```python
from build123d import *

# Parameters (mm, degrees)
SKETCH1_R           = 37.5
BOSS_EXTRUDE1_DEPTH = 28.75
SKETCH2_R           = 31.5
SKETCH2_R_2         = 15.75
BOSS_EXTRUDE2_DEPTH = 6.5
SKETCH3_R           = 6
BOSS_EXTRUDE3_DEPTH = 58.85
SKETCH4_R           = 7.5
BOSS_EXTRUDE4_DEPTH = 4.7
CHAMFER1_SIZE       = 1
SKETCH5_R           = 2.5
CUT_EXTRUDE1_DEPTH  = 8
CHAMFER2_SIZE       = 1


with BuildPart() as part:
    # Sketch1 → Boss-Extrude1 (new body)
    with BuildSketch(Plane(origin=(0, 0, 0), x_dir=(1, 0, 0), z_dir=(0, 1, 0))):
        with Locations(Location((0, 0, 0), (0, 0, 90))):
            Circle(SKETCH1_R)
    extrude(amount=BOSS_EXTRUDE1_DEPTH)

    # Sketch2 → Boss-Extrude2 (add)
    with BuildSketch(Plane(origin=(0, 28.75, 0), x_dir=(1, 0, 0), z_dir=(0, 1, 0))):
        with Locations(Location((0, 0, 0), (0, 0, 90))):
            Circle(SKETCH2_R)
        with Locations(Location((0, 0, 0), (0, 0, 90))):
            Circle(SKETCH2_R_2, mode=Mode.SUBTRACT)
    extrude(amount=BOSS_EXTRUDE2_DEPTH)

    # Sketch3 → Boss-Extrude3 (add)
    with BuildSketch(Plane.XZ):
        with Locations(Location((0, 0, 0), (0, 0, 270))):
            Circle(SKETCH3_R)
    extrude(amount=BOSS_EXTRUDE3_DEPTH)

    # Sketch4 → Boss-Extrude4 (add)
    with BuildSketch(Plane.XZ):
        with Locations(Location((0, 0, 0), (0, 0, 90))):
            Circle(SKETCH4_R)
    extrude(amount=BOSS_EXTRUDE4_DEPTH)

    # Chamfer1
    chamfer1_edges = [part.edges().sort_by_distance(p)[0] for p in [
        (0, 28.75, 37.5),
        (0, 35.25, 31.5),
    ]]
    chamfer(chamfer1_edges, length=CHAMFER1_SIZE)

    # Sketch5 → Cut-Extrude1 (cut)
    with BuildSketch(Plane(origin=(0, 35.25, 0), x_dir=(1, 0, 0), z_dir=(0, 1, 0))):
        with Locations(Location((0, 25, 0), (0, 0, 270))):
            Circle(SKETCH5_R)
        with Locations(Location((25, 0, 0), (0, 0, 270))):
            Circle(SKETCH5_R)
        with Locations(Location((0, -25, 0), (0, 0, 270))):
            Circle(SKETCH5_R)
        with Locations(Location((-25, 0, 0), (0, 0, 270))):
            Circle(SKETCH5_R)
    extrude(amount=-CUT_EXTRUDE1_DEPTH, mode=Mode.SUBTRACT)

    # Chamfer2
    chamfer2_edges = [part.edges().sort_by_distance(p)[0] for p in [
        (0, 35.25, -27.5),
        (25, 35.25, -2.5),
        (0, 35.25, 22.5),
        (-25, 35.25, -2.5),
    ]]
    chamfer(chamfer2_edges, length=CHAMFER2_SIZE)


solid = part.part
```
Check sheet for the modelled part. Datum: model origin and axes. Units: mm. A direction names the side the tool comes from. Round coordinates to 2 decimals unless told otherwise and drop trailing zeros. Order: outer loops, then holes, each group sorted by start corner. A loop starts at its lowest first (then second) coordinate and runs counter-clockwise, first axis right, second up. Notation, with made-up numbers: (84.25, -33.75) -> (118.25, -33.75) arc R28 ccw to (118.25, -13.75) -> close; hole circle Ø7 at (41.25, -7). An arc over 180 degrees is marked (long way). Use CSV: the item, a comma, the result in double quotes.
(1) Depth check by flat-ended pin: pin 1 (2.5 mm diameter, centred on x = -26, z = -0.5, fed in from +Y); pin 2 (4 mm diameter, centred on x = 1, z = 25, fed in from +Y); pin 3 (19 mm diameter, centred on x = 0, z = 0, fed in from +Y). Enter the tip coordinate at first touch or a pass-through.
Worked out:
pin 1,"y = 27.25"
pin 2,"y = 34.75"
pin 3,"y = 28.75"
(2) Cross-section at A-A (y = -46). Record the boundary of the cut face in (x, z).
Worked out:
outline,"circle Ø12 at (0, 0)"
(3) Tool access check on faces 1 (the face through (-6, -4.7, 2)), 2 (the face through (11, 28.75, 30)), 3 (the face through (22.818, 13.681, 29.759)). Record the directions out of +Z, -Z, +X, -X, +Y, -Y that give a thin tool (end or side, any length) a straight path to the whole face; none if there is none.
Worked out:
face 1,"-Y"
face 2,"+Y"
face 3,"+Y, -Y"
(4) Material ranges on line 1 along X through (y, z) = (30, 0); line 2 along Y through (x, z) = (3.5, -15); line 3 along Z through (x, y) = (-30, 14), recorded low to high. Write a range as from..to.
Worked out:
line 1,"-31.5..-27.5, -22.5..-15.75, 15.75..22.5, 27.5..31.5"
line 2,"0..28.75"
line 3,"-22.5..22.5"
(5) Draft check along Z on faces 4 (the face through (-15.616, 31.954, 2.05)), 5 (the face through (8, 0, 1)), 6 (the face through (-31.232, 31.462, 4.101)), 7 (the face through (-25, 27.25, 0)). Enter one of: pulls with the +Z half, pulls with the -Z half, needs draft (parallel to the pull), parting line crosses it, or undercut.
Worked out:
face 4,"undercut"
face 5,"needs draft"
face 6,"parting line crosses it"
face 7,"undercut"
(6) Cross-section at B-B (y = -2). Record the boundary of the cut face in (x, z), and give its area (3 significant figures).
Worked out:
outline,"circle Ø15 at (0, 0)"
area,"177 mm²"
